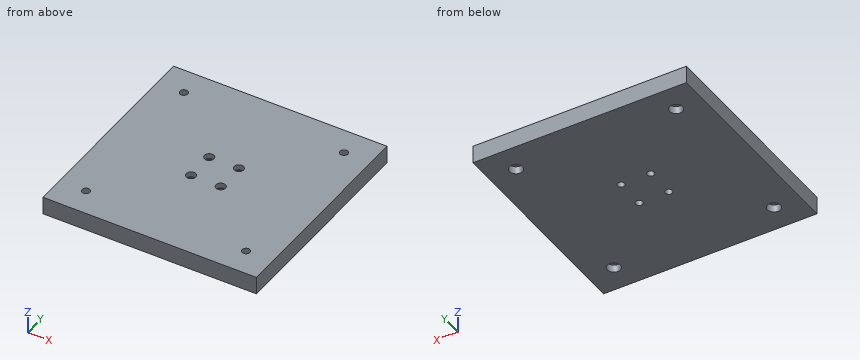
from build123d import *

# Parameters (mm, degrees)
ESQUISSE1_W                                        = 180
ESQUISSE1_H                                        = 180
ESQUISSE1_R                                        = 3
BOSS_EXTRU_1_DEPTH                                 = 15
ESQUISSE6_R                                        = 3
ENL_V_MAT_EXTRU_1_DEPTH                            = 16
CHAMBRAGE_POUR_VIS_T_TE_HEXAGONALE_M41_D           = 4.5
CHAMBRAGE_POUR_VIS_T_TE_HEXAGONALE_M41_CBORE_D     = 8
CHAMBRAGE_POUR_VIS_T_TE_HEXAGONALE_M41_CBORE_DEPTH = 4.4
CHAMBRAGE_POUR_VIS_T_TE_HEXAGONALE_M62_D           = 6.6
CHAMBRAGE_POUR_VIS_T_TE_HEXAGONALE_M62_CBORE_D     = 11
CHAMBRAGE_POUR_VIS_T_TE_HEXAGONALE_M62_CBORE_DEPTH = 6.4


with BuildPart() as part:
    # Esquisse1 → Boss.-Extru.1 (new body)
    with BuildSketch(Plane.XY):
        with Locations((-90, 90)):
            Rectangle(ESQUISSE1_W, ESQUISSE1_H)
        with Locations((-22.5, 22.5)):
            Circle(ESQUISSE1_R, mode=Mode.SUBTRACT)
        with Locations((-157.5, 22.5)):
            Circle(ESQUISSE1_R, mode=Mode.SUBTRACT)
        with Locations((-157.5, 157.5)):
            Circle(ESQUISSE1_R, mode=Mode.SUBTRACT)
        with Locations((-22.5, 157.5)):
            Circle(ESQUISSE1_R, mode=Mode.SUBTRACT)
    extrude(amount=BOSS_EXTRU_1_DEPTH)

    # Esquisse6 → Enlèv. mat.-Extru.1 (cut, through all)
    with BuildSketch(Plane.XY.offset(15)):
        with Locations((-102.5, 77.5)):
            Circle(ESQUISSE6_R)
        with Locations((-77.5, 77.5)):
            Circle(ESQUISSE6_R)
        with Locations((-77.5, 102.5)):
            Circle(ESQUISSE6_R)
        with Locations((-102.5, 102.5)):
            Circle(ESQUISSE6_R)
    extrude(amount=-ENL_V_MAT_EXTRU_1_DEPTH, mode=Mode.SUBTRACT)

    # Chambrage pour vis à tête hexagonale M41 (through all)
    with Locations(Plane.XY.offset(15)):
        with Locations((-102.5, 77.5), (-102.5, 102.5), (-77.5, 102.5), (-77.5, 77.5)):
            CounterBoreHole(CHAMBRAGE_POUR_VIS_T_TE_HEXAGONALE_M41_D / 2, CHAMBRAGE_POUR_VIS_T_TE_HEXAGONALE_M41_CBORE_D / 2, CHAMBRAGE_POUR_VIS_T_TE_HEXAGONALE_M41_CBORE_DEPTH)

    # Chambrage pour vis à tête hexagonale M62 (through all)
    with Locations(Plane(origin=(0, 0, 0), x_dir=(-1, 0, 0), z_dir=(0, 0, -1))):
        with Locations((157.5, 22.5), (22.5, 22.5), (22.5, 157.5), (157.5, 157.5)):
            CounterBoreHole(CHAMBRAGE_POUR_VIS_T_TE_HEXAGONALE_M62_D / 2, CHAMBRAGE_POUR_VIS_T_TE_HEXAGONALE_M62_CBORE_D / 2, CHAMBRAGE_POUR_VIS_T_TE_HEXAGONALE_M62_CBORE_DEPTH)


solid = part.part
The model under review builds one solid part; all positions refer to its coordinate system, in mm. Give positions to 0.01 mm unless a question says otherwise; leave off trailing zeros. Write each loop counter-clockwise with the first axis right and the second up, starting at its lowest first coordinate (ties: lowest second). Pieces come first, ordered by that corner, then holes.
1. Add section A-A, the plane y = 157.5. Write out the cut boundary in (x, z), plus the area to 3 significant figures.
2. Add section B-B, the plane x = -77.5. Write out the cut boundary in (y, z), plus the area to 3 significant figures.
3. Wall thickness on L1, parallel to X at y = 77, z = 2.25; L2, parallel to Y at x = -77.5, z = 3; L3, parallel to Y at x = -157.5, z = 2.5: over which ranges is each line inside the solid? List them lowest first.
4. For P1, Ø5.5, axis at x = -158.5, y = 159.5, coming from the -Z side; P2, Ø7, axis at x = -102.5, y = 102.5, coming from the +Z side, all flat-tipped, find the tip position at first contact; note any pin that passes through.
Worked answers:
1. outline: (-180, 0) - (-163, 0) - (-163, 6.4) - (-160.8, 6.4) - (-160.8, 15) - (-180, 15) - close; (-154.2, 6.4) - (-152, 6.4) - (-152, 0) - (-28, 0) - (-28, 6.4) - (-25.8, 6.4) - (-25.8, 15) - (-154.2, 15) - close; (-19.2, 6.4) - (-17, 6.4) - (-17, 0) - (0, 0) - (0, 15) - (-19.2, 15) - close
1. area: 2,450 mm2
2. outline: (0, 0) - (74.5, 0) - (74.5, 10.6) - (73.5, 10.6) - (73.5, 15) - (0, 15) - close; (80.5, 0) - (99.5, 0) - (99.5, 10.6) - (98.5, 10.6) - (98.5, 15) - (81.5, 15) - (81.5, 10.6) - (80.5, 10.6) - close; (105.5, 0) - (180, 0) - (180, 15) - (106.5, 15) - (106.5, 10.6) - (105.5, 10.6) - close
2. area: 2,500 mm2
3. L1: x = -180 to -105.46, -99.54 to -80.46, -74.54 to 0
3. L2: y = 0 to 74.5, 80.5 to 99.5, 105.5 to 180
3. L3: y = 0 to 17, 28 to 152, 163 to 180
4. P1: stops at z = 6.4
4. P2: stops at z = 10.6
